The model under review builds one solid part; all positions refer to its coordinate system, in mm. Face numbers are marked on the shaded views. A direction names the side the tool comes from. Give positions to 0.01 mm unless a question says otherwise; leave off trailing zeros. Loops run counter-clockwise (first coordinate to the right, second up) from the corner with the lowest first, then second, coordinate; pieces in that order, holes last. Notation, with made-up numbers: M 68.25,-15.5 L 84.25,-15.5 A27 ccw 84.25,16.5 Z; hole C 0.25,65 d11. An arc over 180 degrees is marked long. Write item = value, one per line. Start each with the question number.
1. For the marked faces 1, 2 and 3, list the 3-axis set-ups (+Z, -Z, +X, -X, +Y, -Y) from which the entire face can be reached by the end or side of a thin tool; tool diameter is ignored.
2. We need section A-A on y = 1.1. Give the boundary of the cut face in (x, z), then the cut area to 3 significant figures.
3. We need section C-C on x = 4.5. Give the boundary of the cut face in (y, z), then the cut area to 3 significant figures.
4. We need section B-B on y = 3.4. Give the boundary of the cut face in (x, z).
5. For pin 1 (1.4 mm diameter, centred on y = 1, z = -5, fed in from +X); pin 2 (1.5 mm diameter, centred on y = 0.5, z = -2, fed in from -X); pin 3 (0.9 mm diameter, centred on x = 8, z = -5.5, fed in from -Y), all flat-tipped, find the tip position at first contact; note any pin that passes through.
6. Wall thickness on line 1 along Y through (x, z) = (8, -7.25); line 2 along X through (y, z) = (3.45, -4); line 3 along Y through (x, z) = (13, -4): over which ranges is each line inside the solid? List them lowest first. Write a range as from..to.
7. Draft analysis for pull direction X (two halves, no side actions). For the marked faces 4, 5 and 6, state which applies: pulls with the +X half, pulls with the -X half, needs draft (parallel to the pull), parting line crosses it, or undercut.
from build123d import *

# Parameters (mm, degrees)
SKETCH1_W           = 15.24
SKETCH1_H           = 7.874
BOSS_EXTRUDE1_DEPTH = 2.54
SKETCH2_R           = 3.937
BOSS_EXTRUDE2_DEPTH = 1.524
SKETCH3_R           = 1.397
CUT_EXTRUDE1_DEPTH  = 18.628771143
FILLET1_R           = 3.937
SKETCH4_W           = 3.048
SKETCH4_H           = 7.874
CUT_EXTRUDE2_DEPTH  = 1.27
CHAMFER1_SIZE       = 0.6096


with BuildPart() as part:
    # Sketch1 → Boss-Extrude1 (new body)
    with BuildSketch(Plane(origin=(0, 0, 0), x_dir=(1, 0, 0), z_dir=(0, 1, 0))):
        with Locations((7.62, 3.937)):
            Rectangle(SKETCH1_W, SKETCH1_H)
    extrude(amount=BOSS_EXTRUDE1_DEPTH)

    # Sketch2 → Boss-Extrude2 (add)
    with BuildSketch(Plane(origin=(0, 2.54, 0), x_dir=(1, 0, 0), z_dir=(0, 1, 0))):
        with Locations(Location((7.62, 3.937, 0), (0, 0, 270))):
            Circle(SKETCH2_R)
    extrude(amount=BOSS_EXTRUDE2_DEPTH)

    # Sketch3 → Cut-Extrude1 (cut, through all)
    with BuildSketch(Plane(origin=(0, 4.064, 0), x_dir=(1, 0, 0), z_dir=(0, 1, 0))):
        with Locations(Location((7.62, 3.937, 0), (0, 0, 270))):
            Circle(SKETCH3_R)
    extrude(amount=-CUT_EXTRUDE1_DEPTH, mode=Mode.SUBTRACT)

    # Fillet1
    fillet1_edges = [part.edges().sort_by_distance(p)[0] for p in [
        (15.24, 1.27, -7.874),
        (0, 1.27, 0),
    ]]
    fillet(fillet1_edges, radius=FILLET1_R)

    # Sketch4 → Cut-Extrude2 (cut)
    with BuildSketch(Plane.XZ):
        with Locations((7.62, -3.937)):
            Rectangle(SKETCH4_W, SKETCH4_H)
    extrude(amount=-CUT_EXTRUDE2_DEPTH, mode=Mode.SUBTRACT)

    # Chamfer1
    chamfer1_edges = [part.edges().sort_by_distance(p)[0] for p in [
        (10.2235, 0, -7.874),
        (14.086879398, 0, -6.720879398),
        (15.24, 0, -1.9685),
        (5.0165, 0, 0),
        (1.153120602, 0, -1.153120602),
        (0, 0, -5.9055),
    ]]
    chamfer(chamfer1_edges, length=CHAMFER1_SIZE)


solid = part.part
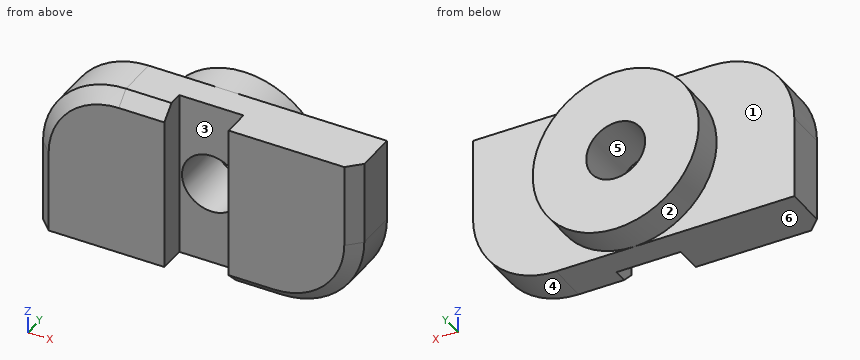
Final values:
q1.face_1 = -X, +Y
q1.face_2 = +Y
q1.face_3 = +Z, -Z, -Y
q2.outline = M 0,-7.87 L 6.1,-7.87 L 6.1,0 L 3.94,0 A3.94 ccw 0,-3.94 Z; M 9.14,-7.87 L 11.3,-7.87 A3.94 ccw 15.24,-3.94 L 15.24,0 L 9.14,0 Z
q2.area = 89.3 mm²
q3.outline = M 0,-7.87 L 2.54,-7.87 L 2.54,-6.34 L 4.06,-6.34 L 4.06,-1.54 L 2.54,-1.54 L 2.54,0 L 0.61,0 L 0,-0.61 Z
q3.area = 27.1 mm²
q4.outline = C 7.62,-3.94 d7.87; hole C 7.62,-3.94 d2.79
q5.pin_1 = 15.22
q5.pin_2 = 0.19
q5.pin_3 = 1.27
q6.line_1 = 1.27..4.06
q6.line_2 = 3.68..6.22, 9.02..11.56
q6.line_3 = 0..2.54
q7.face_4 = pulls with the +X half
q7.face_5 = undercut
q7.face_6 = needs draft
